Autodesk Inventor part; units mm, degrees
ref_plane "YZ Plane" through (0, 0, 0) normal (1, 0, 0) x (0, 1, 0)
ref_plane "XZ Plane" through (0, 0, 0) normal (0, 1, 0) x (-1, 0, 0)
ref_plane "XY Plane" through (0, 0, 0) normal (0, 0, 1) x (1, 0, 0)
sketch "Sketch1" plane through (0, 0, 0) normal (1, 0, 0) x (0, 1, 0)
  line L0 (0, 0) -> (0, 32.5)
  line L1 (0, 0) -> (40.5, 0)
  line L2 (23, 18.5) -> (28.5, 18.5)
  line L3 (28.5, 18.5) -> (28.5, 14.75)
  line L4 (28.5, 14.75) -> (40.5, 14.75)
  line L5 (40.5, 14.75) -> (40.5, 0)
  line L6 (0, 32.5) -> (9, 32.5)
  line L7 (9, 32.5) -> (9, 22.25)
  line L8 (9, 22.25) -> (12, 22.25)
  line L9 (12, 22.25) -> (23, 18.5)
  dimension "d0" = 32.5
  dimension "d1" = 12
  dimension "d2" = 14.75
  dimension "d4" = 18.5
  dimension "d5" = 5.5
  dimension "d6" = 14
  dimension "d7" = 3
  dimension "d8" = 9
  dimension "d9" = 22.25
revolve "Revolution1" add sketch "Sketch1" angle 360 about axis through (0, 0, 0) along (0, 1, 0)
sketch "Sketch2" plane through (0, 40.5, 0) normal (0, 1, 0) x (1, 0, 0)
  circle A0 centre (0, 0) radius 14.75
  line L0 (0, 0) -> (11, 0) construction
  dimension "d11" = 11
hole "Hole1" at (11, 40.5, 0) direction (0, -1, 0) diameter 4.5 end through all
hole "Hole2" at (0, 40.5, 0) direction (0, -1, 0) diameter 10 end through all
sketch "Sketch3" plane through (0, 0, 0) normal (0, -1, 0) x (1, 0, 0)
  line L0 (15.3301, 0) -> (13.1651, -3.75)
  line L1 (13.1651, -3.75) -> (8.8349, -3.75)
  line L2 (8.8349, -3.75) -> (6.6699, 0)
  line L3 (6.6699, 0) -> (8.8349, 3.75)
  line L4 (8.8349, 3.75) -> (13.1651, 3.75)
  line L5 (13.1651, 3.75) -> (15.3301, 0)
  circle A0 centre (11, 0) radius 2.25
  circle A1 centre (0, 0) radius 32.5
  line L6 (11, 0) -> (0, 0) construction
  line L7 (0, 0) -> (10.253, -10.253) construction
  point P0 (11, 0)
  dimension "d31" = 7.5
  dimension "d37" = 14.5
  dimension "d38" = 45
extrude "Extrusion1" cut sketch "Sketch3" against normal blind 8 contours L0 L1 L2 L3 L4 L5 | A0
hole "Hole3" at (10.253, 0, -10.253) direction (0, 1, 0) diameter 2 depth 15 tip angle 118
pattern_circular "Circular Pattern2" count 4 over 360 about axis through (0, -10, 0) along (0, 1, 0) of "Extrusion1", "Hole1", "Hole3"
sketch "Sketch4" plane through (0, 0, 0) normal (0, -1, 0) x (1, 0, 0)
  line L0 (0, -6.6699) -> (3.75, -8.8349)
  line L1 (3.75, -8.8349) -> (3.75, -13.1651)
  circle A0 centre (10.253, -10.253) radius 1
  line L2 (13.1651, -3.75) -> (8.8349, -3.75)
  line L3 (8.8349, -3.75) -> (6.6699, 0)
  line L4 (8.8349, 3.75) -> (13.1651, 3.75)
  circle A1 centre (0, 0) radius 32.5
  line L5 (0, -6.6699) -> (0, 0)
  line L6 (0, 0) -> (6.6699, 0)
  line L7 (3.75, -13.1651) -> (10.5296, -11.214)
  line L8 (13.1651, -3.75) -> (11.214, -10.5296)
extrude "Extrusion2" cut sketch "Sketch4" against normal up to surface (8 mm away) contours L5 L6 L3 L2 L8 A0 L7 L1 L0
properties part number "stand_coupler1" material "ABS Plastic"
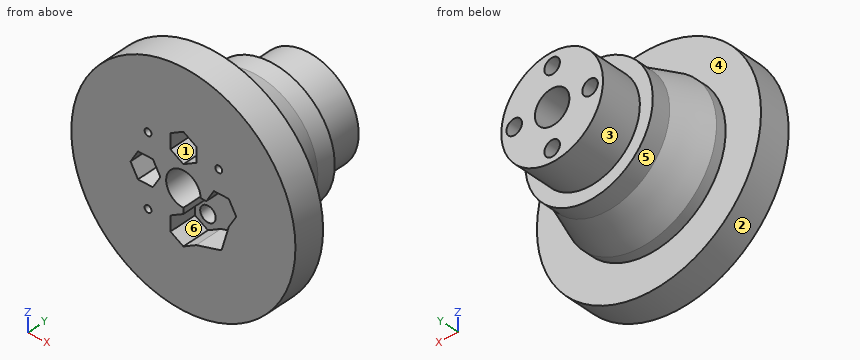
Can you work these out from the model? Positions are in its coordinate system, mm. Face numbers are marked on the shaded views. A direction names the side the tool comes from. Coordinates: 2 decimals unless noted, no trailing zeros. Write each loop counter-clockwise with the first axis right and the second up, starting at its lowest first coordinate (ties: lowest second). Pieces come first, ordered by that corner, then holes.
Q1. Imagine slicing it at D-D, the plane z = 28.5. List the corners of the cut face in (x, y) for me.
Results found:
outline: (-15.62, 0) - (15.62, 0) - (15.62, 9) - (-15.62, 9) - close
Q2. Imagine slicing it at C-C, the plane x = -23.5. List the corners of the cut face in (y, z) for me, plus the area to 3 significant figures.
Results found:
outline: (0, -22.45) - (9, -22.45) - (9, 22.45) - (0, 22.45) - close
area: 404 mm2
Q3. Which directions (+Z, -Z, +X, -X, +Y, -Y) give clear straight access to the entire face, cutting with the end or side of a thin tool? Please do the marked faces 1, 2 and 3.
Results found:
face 1: -Y
face 2: +Y, -Y
face 3: +Y
Q4. Imagine slicing it at B-B, the plane y = 30. List the corners of the cut face in (x, z) for me, plus the area to 3 significant figures.
Results found:
outline: circle Ø29.5 at (0, 0); hole circle Ø4.5 at (-11, 0); hole circle Ø10 at (0, 0); hole circle Ø4.5 at (0, -11); hole circle Ø4.5 at (0, 11); hole circle Ø4.5 at (11, 0)
area: 541 mm2
Q5. Imagine slicing it at A-A, the plane y = 7. Count the separate pieces of the cut face and the enclosed holes in it, plus the area to 3 significant figures.
Results found:
separate pieces: 1
enclosed holes: 6
area: 2,940 mm2
Q6. For P1, Ø21, axis at x = 3.5, z = -3.5, coming from the -Y side; P2, Ø2, axis at y = 6, z = -6, coming from the -X side; P3, Ø5, axis at x = -6, y = 6, coming from the +Z side; P4, Ø1.3, axis at x = 10, y = 3, coming from the -Z side, each with a flat end and sliding along its axis, tell me the tip position at first contact or that it passes through.
Results found:
P1: stops at y = 0
P2: stops at x = -32.11
P3: stops at z = 32.31
P4: stops at z = -31.13
Q7. Please list where these lines run through material, in increasing order: L1, parallel to X at y = 29, z = 0; L2, parallel to X at y = 25, z = 0; L3, parallel to Y at x = -3.5, z = -25.
Results found:
L1: x = -14.75 to -13.25, -8.75 to -5, 5 to 8.75, 13.25 to 14.75
L2: x = -18.5 to -13.25, -8.75 to -5, 5 to 8.75, 13.25 to 18.5
L3: y = 0 to 9
Q8. If we mould it in two halves opening along X, with no side actions, what happens to the marked faces 4, 5 and 6? For each: +X half, -X half, draft (parallel to the pull), parting line (faces both ways), or undercut.
Results found:
face 4: draft
face 5: parting line
face 6: undercut
